Autodesk Fusion 360 part; units mm, degrees
sketch "Sketch1" plane through (0, 0, 0) normal (0, 1, 0) x (1, 0, 0)
  line L0 (1.5, -2) -> (-1.5, -2)
  line L1 (-2, -1.5) -> (-2, 1.5)
  line L2 (-1.5, 2) -> (1.5, 2)
  line L3 (2, 1.5) -> (2, -1.5)
  line L4 (2, -2) -> (-2, 2) construction
  line L5 (-2, -2) -> (2, 2) construction
  line L6 (-1.5, -3) -> (1.5858, -3)
  line L7 (3, -1.5858) -> (3, 1.5)
  line L8 (1.5, 3) -> (-1.5, 3)
  line L9 (-3, 1.5) -> (-3, -1.5)
  line L10 (-3, -3) -> (3, 3) construction
  line L11 (3, -3) -> (-2.9939, 2.9939) construction
  arc A0 (-1.5, 2) -> (-2, 1.5) centre (-1.5, 1.5) ccw
  arc A1 (-2, -1.5) -> (-1.5, -2) centre (-1.5, -1.5) ccw
  arc A2 (1.5, -2) -> (2, -1.5) centre (1.5, -1.5) ccw
  arc A3 (2, 1.5) -> (1.5, 2) centre (1.5, 1.5) ccw
  arc A4 (-1.5, 3) -> (-3, 1.5) centre (-1.5, 1.5) ccw
  arc A5 (-3, -1.5) -> (-1.5, -3) centre (-1.5, -1.5) ccw
  arc A6 (3, 1.5) -> (1.5, 3) centre (1.5, 1.5) ccw
  line L12 (3.7071, -2.2929) -> (2.2929, -3.7071)
  line L13 (2.2929, -3.7071) -> (1.5858, -3)
  line L14 (3, -1.5858) -> (3.7071, -2.2929)
  dimension "d1" = 4
  dimension "d2" = 4
  dimension "d3" = 0.5
  dimension "d4" = 6
  dimension "d5" = 6
  dimension "d6" = 1.5
  dimension "d7" = 2
  dimension "d31" = 2
  dimension "d32" = 3
extrude "Extrude1" add sketch "Sketch1" along normal blind 2.5
sketch "Sketch2" plane through (3, 0, 3) normal (0.7071, 0, 0.7071) x (0.7071, 0, -0.7071)
  line L0 (-1, 0) -> (1, 0)
  line L1 (1, 0) -> (1, 2.5)
  line L2 (1, 2.5) -> (-1, 2.5)
  line L3 (-1, 2.5) -> (-1, 0)
  circle A0 centre (0, 1.5) radius 0.595
  dimension "d10" = 1.19
  dimension "d11" = 1.5
extrude "Extrude2" cut sketch "Sketch2" along direction (-0.70231, 0, -0.711871) blind 3.4 contours A0
sketch "Sketch4" plane through (0, 0, 0) normal (0, -1, 0) x (1, 0, 0)
  arc A0 (2, 1.5) -> (1.5, 2) centre (1.5, 1.5) ccw
  line L0 (2, 1.5) -> (2, -1.5)
  arc A1 (1.5, -2) -> (2, -1.5) centre (1.5, -1.5) ccw
  line L1 (1.5, -2) -> (-1.5, -2)
  arc A2 (-2, -1.5) -> (-1.5, -2) centre (-1.5, -1.5) ccw
  line L2 (-2, -1.5) -> (-2, 1.5)
  arc A3 (-1.5, 2) -> (-2, 1.5) centre (-1.5, 1.5) ccw
  line L3 (-1.5, 2) -> (1.5, 2)
  line L4 (3, 1.5858) -> (3.7071, 2.2929)
  line L5 (3.7071, 2.2929) -> (2.2929, 3.7071)
  line L6 (2.2929, 3.7071) -> (1.5858, 3)
  line L7 (1.5858, 3) -> (-1.5, 3)
  arc A4 (-1.5, 3) -> (-3, 1.5) centre (-1.5, 1.5) ccw
  line L8 (-3, 1.5) -> (-3, -1.5)
  arc A5 (-3, -1.5) -> (-1.5, -3) centre (-1.5, -1.5) ccw
  line L9 (-1.5, -3) -> (1.5, -3)
  arc A6 (1.5, -3) -> (3, -1.5) centre (1.5, -1.5) ccw
  line L10 (3, -1.5) -> (3, 1.5858)
  line L11 (-0.7071, 5) -> (0.7929, 5)
  line L12 (0.7929, 5) -> (0.7929, 3)
  line L13 (-0.7071, 3) -> (-0.7071, 5)
  line L14 (-0.7071, 5) -> (0.6239, 1.4506) construction
  line L15 (0.7929, 5) -> (-0.5381, 1.4506) construction
  line L16 (-5, -0.7071) -> (-1.4506, 0.6239) construction
  line L17 (-5, -0.7071) -> (-5, 0.7929)
  line L18 (-5, 0.7929) -> (-1.4506, -0.5381) construction
  line L19 (-3, -0.7071) -> (-5, -0.7071)
  line L20 (-5, 0.7929) -> (-3, 0.7929)
  line L21 (0.7071, -5) -> (-0.6239, -1.4506) construction
  line L22 (0.7071, -5) -> (-0.7929, -5)
  line L23 (-0.7929, -5) -> (0.5381, -1.4506) construction
  line L24 (0.7071, -3) -> (0.7071, -5)
  line L25 (-0.7929, -5) -> (-0.7929, -3)
  line L26 (5, 0.7071) -> (1.4506, -0.6239) construction
  line L27 (5, 0.7071) -> (5, -0.7929)
  line L28 (5, -0.7929) -> (1.4506, 0.5381) construction
  line L29 (3, 0.7071) -> (5, 0.7071)
  line L30 (5, -0.7929) -> (3, -0.7929)
  line L31 (0.0429, 3) -> (0.0429, 5) construction
  line L32 (0.6239, 1.4506) -> (-0.5381, 1.4506)
  point P0 (0.0429, 3)
  point P1 (-3, 0.0429)
  point P2 (-0.0429, -3)
  point P3 (3, -0.0429)
  dimension "d26" = 360
  dimension "d29" = 1.5
  dimension "d30" = 2
extrude "Extrude4" add sketch "Sketch4" against normal blind 1 contours L10 L27 L29 L30 | L7 L11 L12 L13 | L9 L22 L24 L25 | L8 L17 L19 L20
fillet "Fillet2" radius 0.5 8 edges at (3, 0.5, 0.7071) (0.7929, 0.5, 3) (3, 0.5, -0.7929) (0.7071, 0.5, -3) (-0.7929, 0.5, -3) (-3, 0.5, -0.7071) (-0.7071, 0.5, 3) (-3, 0.5, 0.7929)
fillet "Fillet3" radius 0.5 2 edges at (1.5858, 1.25, 3) (3, 1.25, 1.5858)
extrude "Extrude5" add 1 faces at (2.3333, 2.5, 0.4596) along direction (0, 1, 0) blind 0.5
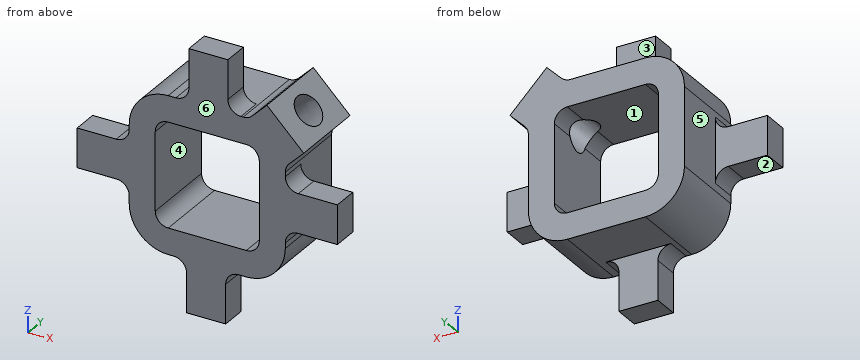
Geometry check sheet. Reference: the model listing, model coordinates, mm. Face numbers are marked on the shaded views. A direction names the side the tool comes from. Round coordinates to 2 decimals unless told otherwise and drop trailing zeros. Order: outer loops, then holes, each group sorted by start corner. A loop starts at its lowest first (then second) coordinate and runs counter-clockwise, first axis right, second up. Notation, with made-up numbers: (71.25, 33) -> (113.25, 33) arc R29 cw to (113.25, 63) -> close; hole circle Ø5 at (-32.5, -38.5). An arc over 180 degrees is marked (long way). Return JSON: item names as keys, results as strings. Group by question number.
Q1. Gauge pin test, flat ends, axial feed: pin 1 (1.1 mm diameter, centred on y = 0.5, z = 4.5, fed in from +X); pin 2 (1 mm diameter, centred on x = -0.5, z = -4, fed in from +Y); pin 3 (0.5 mm diameter, centred on x = -4.5, y = 0.5, fed in from -Z). Record the tip position at first contact, or that the pin passes through.
Q2. Material ranges on probe 1 along Z at (x, y) = (-1.25, 1.6); probe 2 along X at (y, z) = (1.6, 1.5), recorded low to high. Write a range as from..to.
Q3. Section check C-C, the plane y = 2.6. Record the boundary of the cut face in (x, z), plus the area to 3 significant figures.
Q4. Section check D-D, the plane x = -4.5. Record the boundary of the cut face in (y, z), plus the area to 3 significant figures.
Q5. Section check B-B, the plane z = -0.25. Record the boundary of the cut face in (x, y).
Q6. Tool access check on the marked faces 1, 2 and 3. Record the directions out of +Z, -Z, +X, -X, +Y, -Y that give a thin tool (end or side, any length) a straight path to the whole face; none if there is none.
Q7. Section check A-A, the plane x = 0. Record the boundary of the cut face in (y, z).
Q8. Release check for a two-part mould opening along X. For the marked faces 4, 5 and 6 record: released by +X, released by -X, zero draft, split by the parting line, or undercut.
Numbers:
{
 "1": {"pin 1": "x = 0.79", "pin 2": "y = 1", "pin 3": "z = -0.71"},
 "2": {"probe 1": "-3..-2, 2..3", "probe 2": "-3..-2, 2.34..3.01"},
 "3": {"outline": "(-3, -1.5) arc R1.5 ccw to (-1.5, -3) -> (1.5, -3) arc R1.5 ccw to (3, -1.5) -> (3, 1.38) arc R0.5 cw to (3.15, 1.73) -> (3.71, 2.29) -> (2.29, 3.71) -> (1.73, 3.15) arc R0.5 cw to (1.38, 3) -> (-1.5, 3) arc R1.5 ccw to (-3, 1.5) -> close; hole (-2, -1.5) arc R0.5 ccw to (-1.5, -2) -> (1.5, -2) arc R0.5 ccw to (2, -1.5) -> (2, 1.5) arc R0.5 ccw to (1.5, 2) -> (-1.5, 2) arc R0.5 ccw to (-2, 1.5) -> close", "area": "19.8 mm^2"},
 "4": {"outline": "(0, -0.71) -> (1, -0.71) -> (1, 0.79) -> (0, 0.79) -> close", "area": "1.50 mm^2"},
 "5": {"outline": "(-5, 0) -> (-2, 0) -> (-2, 3) -> (-3, 3) -> (-3, 1) -> (-5, 1) -> close; (2, 0) -> (5, 0) -> (5, 1) -> (3, 1) -> (3, 3) -> (2, 3) -> close"},
 "6": {"face 1": "+Y, -Y", "face 2": "-Z, -X, +Y, -Y", "face 3": "+Z, -X, +Y"},
 "7": {"outline": "(0, -5) -> (1, -5) -> (1, -3) -> (3, -3) -> (3, -2) -> (0, -2) -> close; (0, 2) -> (3, 2) -> (3, 3) -> (1, 3) -> (1, 5) -> (0, 5) -> close"},
 "8": {"face 4": "undercut", "face 5": "released by -X", "face 6": "zero draft"}
}
